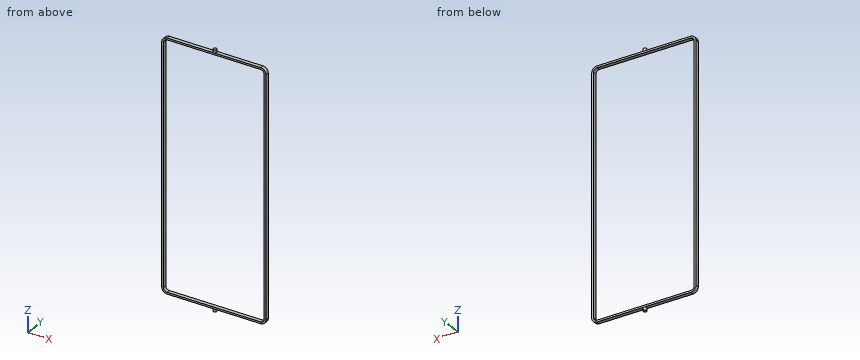
Autodesk Inventor part; units mm, degrees
ref_plane "YZ Plane" through (0, 0, 0) normal (1, 0, 0) x (0, 1, 0)
ref_plane "XZ Plane" through (0, 0, 0) normal (0, 1, 0) x (-1, 0, 0)
ref_plane "XY Plane" through (0, 0, 0) normal (0, 0, 1) x (1, 0, 0)
sketch "Sketch1" plane through (0, 0, 0) normal (0, 1, 0) x (-1, 0, 0)
  line L0 (-3.175, 0) -> (-85.725, 0)
  line L1 (-88.9, -3.175) -> (-88.9, -213.3854)
  line L2 (-85.725, -216.5604) -> (-3.175, -216.5604)
  line L3 (0, -213.3854) -> (0, -3.175)
  arc A0 (0, -3.175) -> (-3.175, 0) centre (-3.175, -3.175) ccw
  arc A1 (-85.725, 0) -> (-88.9, -3.175) centre (-85.725, -3.175) ccw
  arc A2 (-88.9, -213.3854) -> (-85.725, -216.5604) centre (-85.725, -213.3854) ccw
  arc A3 (-3.175, -216.5604) -> (0, -213.3854) centre (-3.175, -213.3854) ccw
  line L4 (1.5875, -3.175) -> (1.5875, -213.3854)
  arc A4 (-3.175, -218.1479) -> (1.5875, -213.3854) centre (-3.175, -213.3854) ccw
  line L5 (-3.175, -218.1479) -> (-85.725, -218.1479)
  arc A5 (-90.4875, -213.3854) -> (-85.725, -218.1479) centre (-85.725, -213.3854) ccw
  line L6 (-90.4875, -213.3854) -> (-90.4875, -3.175)
  arc A6 (-85.725, 1.5875) -> (-90.4875, -3.175) centre (-85.725, -3.175) ccw
  line L7 (-85.725, 1.5875) -> (-3.175, 1.5875)
  arc A7 (1.5875, -3.175) -> (-3.175, 1.5875) centre (-3.175, -3.175) ccw
  point P0 (0, 0)
  point P1 (-88.9, -216.5604)
  point P2 (-88.9, 0)
  point P3 (0, -216.5604)
  dimension "d0" = 88.9
  dimension "d1" = 216.5604
  dimension "d2" = 3.175
extrude "Extrusion2" add sketch "Sketch1" along normal blind 3.175
sketch "Sketch4" plane through (3.175, 0, 1.5875) normal (0, 0, 1) x (1, 0, 0)
  circle A0 centre (41.275, 1.5875) radius 1.5875
  line L0 (0, 0) -> (0, 3.175)
  line L1 (0, 0) -> (82.55, 0)
  point P0 (-3.175, 0)
  dimension "d11" = 3.175
  dimension "d12" = 41.275
  dimension "d13" = 1.5875
extrude "Extrusion3" add sketch "Sketch4" along normal blind 2.54
sketch "Sketch5" plane through (85.725, 0, -218.1479) normal (0, 0, -1) x (-1, 0, 0)
  arc A0 (41.275, 0) -> (41.275, 3.175) centre (41.275, 1.5875) ccw
  circle A1 centre (41.275, 1.5875) radius 1.5875
  point P0 (85.725, 0)
  point P1 (41.275, 3.175)
  point P2 (41.275, 0)
extrude "Extrusion4" add sketch "Sketch5" along normal blind 2.54
properties part number "30t_8.5_in"
Model file for the job. Use its own axes, mm. Give positions to 0.01 mm unless a question says otherwise; leave off trailing zeros. Loops run counter-clockwise (first coordinate to the right, second up) from the corner with the lowest first, then second, coordinate; pieces in that order, holes last. Notation, with made-up numbers: (88.5, 14) -> (125.5, 14) arc R11 ccw to (125.5, 26) -> close; hole circle Ø3 at (88.5, 19.5). An arc over 180 degrees is marked (long way). Use a Markdown table: item, result. Add a question column.
(1) Slice it at A-A on z = -114.5. List the corners of the cut face in (x, y) (1 decimal), and give its area (3 significant figures).
(2) Drop flat-ended pins along their axis: pin 1 Ø1.5 at (x, y) = (52, 1.5) entering from +Z; pin 2 Ø1 at (x, y) = (26, 2) entering from -Z. Give the stop position or say it passes through.
(3) Wall check: line 1 along X through (y, z) = (2.4, -179); line 2 along Z through (x, y) = (7, 2). Give the ranges that are in metal, low to high.
(4) Slice it at B-B on x = 68.5. List the corners of the cut face in (y, z) (1 decimal).
Filled sheet:
| question | item | result |
|---|---|---|
| 1 | outline | (-1.6, 0) -> (0, 0) -> (0, 3.2) -> (-1.6, 3.2) -> close; (88.9, 0) -> (90.5, 0) -> (90.5, 3.2) -> (88.9, 3.2) -> close |
| 1 | area | 10.1 mm2 |
| 2 | pin 1 | z = 1.59 |
| 2 | pin 2 | z = -218.15 |
| 3 | line 1 | -1.59 to 0, 88.9 to 90.49 |
| 3 | line 2 | -218.15 to -216.56, 0 to 1.59 |
| 4 | outline | (0, -218.1) -> (3.2, -218.1) -> (3.2, -216.6) -> (0, -216.6) -> close; (0, 0) -> (3.2, 0) -> (3.2, 1.6) -> (0, 1.6) -> close |
